Geometry: final body of the model. Coordinates: model frame, mm. A direction names the side the tool comes from. Give positions to 0.01 mm unless a question says otherwise; leave off trailing zeros. Write each loop counter-clockwise with the first axis right and the second up, starting at its lowest first coordinate (ties: lowest second). Pieces come first, ordered by that corner, then holes.
```python
from build123d import *

# Parameters (mm, degrees)
F1_DEPTH     = 12.5
F2_DEPTH     = 12.5
F3_DEPTH     = 12.5
F6_DEPTH     = 7.5
F5_R         = 3.429
F7_DEPTH     = 3
F8_T4_DEPTH  = 66.159380005
F8_S5_R      = 15.125
F8_T6_DEPTH  = 35
F8_T10_DEPTH = 66.159380005
F8_S11_R     = 15.125
F8_T12_DEPTH = 35
F8_T16_DEPTH = 66.159380005
F8_S17_R     = 15.125
F8_T18_DEPTH = 35
F8_T22_DEPTH = 66.159380005
F8_S23_R     = 15.125
F8_T24_DEPTH = 35
F9_T1_DEPTH  = 22.0465191056


# Not quite as in the source:
# - a fillet or chamfer that OpenCascade refuses, or shapes differently, is made with other operations: its cross-section is extruded or revolved along the edge and cut away or added


with BuildPart() as f1:
    # F0 (on Front) → F1 (new body, symmetric)
    with BuildSketch(Plane.XZ):
        with BuildLine():
            Line((-6.3651329838, -12.125), (-6.3651329838, -13.7204485021))
            ThreePointArc((-6.3651329838, -13.7204485021), (0, -15.125), (6.3651329838, -13.7204485021))
            Line((6.3651329838, -13.7204485021), (6.3651329838, -12.125))
            Line((6.3651329838, -12.125), (0, -12.125))
            Line((0, -12.125), (-6.3651329838, -12.125))
        make_face()
        with BuildLine():
            ThreePointArc((6.3651329838, 13.7204485021), (3.2591288258, 14.7696887001), (0, 15.125))
            ThreePointArc((0, 15.125), (-3.2591288258, 14.7696887001), (-6.3651329838, 13.7204485021))
            Line((-6.3651329838, 13.7204485021), (-6.3651329838, 12.125))
            Line((-6.3651329838, 12.125), (0, 12.125))
            Line((0, 12.125), (6.3651329838, 12.125))
            Line((6.3651329838, 12.125), (6.3651329838, 13.7204485021))
        make_face()
        with BuildLine():
            ThreePointArc((15.125, 0), (12.7482991293, 8.1391949424), (6.3651329838, 13.7204485021))
            Line((6.3651329838, 13.7204485021), (6.3651329838, 12.125))
            Line((6.3651329838, 12.125), (0, 12.125))
            ThreePointArc((0, 12.125), (8.5736697219, 8.5736697219), (12.125, 0))
            ThreePointArc((12.125, 0), (8.5736697219, -8.5736697219), (0, -12.125))
            Line((0, -12.125), (6.3651329838, -12.125))
            Line((6.3651329838, -12.125), (6.3651329838, -13.7204485021))
            ThreePointArc((6.3651329838, -13.7204485021), (12.7482991293, -8.1391949424), (15.125, 0))
        make_face()
        with BuildLine():
            Line((-6.3651329838, 12.125), (-6.3651329838, 13.7204485021))
            ThreePointArc((-6.3651329838, 13.7204485021), (-15.125, 0), (-6.3651329838, -13.7204485021))
            Line((-6.3651329838, -13.7204485021), (-6.3651329838, -12.125))
            Line((-6.3651329838, -12.125), (0, -12.125))
            ThreePointArc((0, -12.125), (-12.125, 0), (0, 12.125))
            Line((0, 12.125), (-6.3651329838, 12.125))
        make_face()
    extrude(amount=F1_DEPTH, both=True)

    # F0 (on Front) → F2 (join, through all)
    with BuildSketch(Plane.XZ):
        with BuildLine():
            ThreePointArc((6.3651329838, -13.7204485021), (0, -15.125), (-6.3651329838, -13.7204485021))
            Line((-6.3651329838, -13.7204485021), (-6.3651329838, -54.875))
            Line((-6.3651329838, -54.875), (6.3651329838, -54.875))
            Line((6.3651329838, -54.875), (6.3651329838, -13.7204485021))
        make_face()
    extrude(amount=F2_DEPTH)

    # F0 (on Front) → F3 (join, through all)
    with BuildSketch(Plane.XZ):
        with BuildLine():
            Line((6.3651329838, 15.125), (0, 15.125))
            ThreePointArc((0, 15.125), (3.2591288258, 14.7696887001), (6.3651329838, 13.7204485021))
            Line((6.3651329838, 13.7204485021), (6.3651329838, 15.125))
        make_face()
        with BuildLine():
            Line((0, 15.125), (-6.3651329838, 15.125))
            Line((-6.3651329838, 15.125), (-6.3651329838, 13.7204485021))
            ThreePointArc((-6.3651329838, 13.7204485021), (-3.2591288258, 14.7696887001), (0, 15.125))
        make_face()
    extrude(amount=F3_DEPTH)

    # F4 (on face) → F6 (join)
    with BuildSketch(Plane.XY.offset(15.125)):
        Polygon((1.7145000001, -9.2196011096), (3.4290000001, -6.25), (1.7144999999, -3.2803988905), (-1.7145, -3.2803988907), (-3.4289999999, -6.25), (-1.7145000001, -9.2196011096), align=None)
    extrude(amount=F6_DEPTH)

    # F5 (on face) → F7 (join)
    with BuildSketch(Plane(origin=(0, 0, -54.875), x_dir=(1, 0, 0), z_dir=(0, 0, -1))):
        with Locations((0, 6.2500000003)):
            Circle(F5_R)
    extrude(amount=F7_DEPTH)

    # F8: fillet of radius 5 on 6 edges, made by hand


with BuildPart() as f8_tool2:
    # F8_s3 → F8_t4 (new body)
    with BuildSketch(Plane.XY.offset(-67.3774142536)):
        with BuildLine():
            ThreePointArc((1.3641672983, 0.0004), (4.9006668897, -1.4644660941), (6.3655329838, -5.0009656854))
            Line((6.3655329838, -5.0009656854), (6.8656695523, -5.0009656854))
            ThreePointArc((6.8656695523, -5.0009656854), (6.8652695523, -2.5004828427), (6.8652695523, 0))
            Line((6.8652695523, 0), (6.3651329838, 0.5001365685))
            ThreePointArc((6.3651329838, 0.5001365685), (3.8646501411, 0.5001365685), (1.3641672983, 0.5005365685))
            Line((1.3641672983, 0.5005365685), (1.3641672983, 0.0004))
        make_face()
    extrude(amount=F8_T4_DEPTH)

    # F8_s5 → F8_t6 (cut, symmetric)
    with BuildSketch(Plane.XZ.offset(2.3)):
        Circle(F8_S5_R)
    extrude(amount=F8_T6_DEPTH, both=True, mode=Mode.SUBTRACT)


with BuildPart() as f1_1:
    add(f1.part)

    # F8_t1: cut F8_tool2
    add(f8_tool2.part, mode=Mode.SUBTRACT)


with BuildPart() as f8_tool8:
    # F8_s9 → F8_t10 (new body)
    with BuildSketch(Plane.XY.offset(-1.2180342485)):
        with BuildLine():
            ThreePointArc((-6.3655329838, -5.0009656854), (-4.9006668897, -1.4644660941), (-1.3641672983, 0.0004))
            Line((-1.3641672983, 0.0004), (-1.3641672983, 0.5005365685))
            ThreePointArc((-1.3641672983, 0.5005365685), (-3.8646501411, 0.5001365685), (-6.3651329838, 0.5001365685))
            Line((-6.3651329838, 0.5001365685), (-6.8652695523, 0))
            ThreePointArc((-6.8652695523, 0), (-6.8652695523, -2.5004828427), (-6.8656695523, -5.0009656854))
            Line((-6.8656695523, -5.0009656854), (-6.3655329838, -5.0009656854))
        make_face()
    extrude(amount=-F8_T10_DEPTH)

    # F8_s11 → F8_t12 (cut, symmetric)
    with BuildSketch(Plane.XZ.offset(2.3)):
        Circle(F8_S11_R)
    extrude(amount=F8_T12_DEPTH, both=True, mode=Mode.SUBTRACT)


with BuildPart() as f1_2:
    add(f1_1.part)

    # F8_t7: cut F8_tool8
    add(f8_tool8.part, mode=Mode.SUBTRACT)


with BuildPart() as f8_tool14:
    # F8_s15 → F8_t16 (new body)
    with BuildSketch(Plane.XY.offset(-67.3774142536)):
        with BuildLine():
            ThreePointArc((1.3641672983, -12.5004), (4.9006668897, -11.0355339059), (6.3655329838, -7.4990343146))
            Line((6.3655329838, -7.4990343146), (6.8656695523, -7.4990343146))
            ThreePointArc((6.8656695523, -7.4990343146), (6.8652695523, -9.9995171573), (6.8652695523, -12.5))
            Line((6.8652695523, -12.5), (6.3651329838, -13.0001365685))
            ThreePointArc((6.3651329838, -13.0001365685), (3.8646501411, -13.0001365685), (1.3641672983, -13.0005365685))
            Line((1.3641672983, -13.0005365685), (1.3641672983, -12.5004))
        make_face()
    extrude(amount=F8_T16_DEPTH)

    # F8_s17 → F8_t18 (cut, symmetric)
    with BuildSketch(Plane.XZ.offset(10.2)):
        Circle(F8_S17_R)
    extrude(amount=F8_T18_DEPTH, both=True, mode=Mode.SUBTRACT)


with BuildPart() as f1_3:
    add(f1_2.part)

    # F8_t13: cut F8_tool14
    add(f8_tool14.part, mode=Mode.SUBTRACT)


with BuildPart() as f8_tool20:
    # F8_s21 → F8_t22 (new body)
    with BuildSketch(Plane.XY.offset(-1.2180342485)):
        with BuildLine():
            ThreePointArc((-1.3641672983, -12.5004), (-4.9006668897, -11.0355339059), (-6.3655329838, -7.4990343146))
            Line((-6.3655329838, -7.4990343146), (-6.8656695523, -7.4990343146))
            ThreePointArc((-6.8656695523, -7.4990343146), (-6.8652695523, -9.9995171573), (-6.8652695523, -12.5))
            Line((-6.8652695523, -12.5), (-6.3651329838, -13.0001365685))
            ThreePointArc((-6.3651329838, -13.0001365685), (-3.8646501411, -13.0001365685), (-1.3641672983, -13.0005365685))
            Line((-1.3641672983, -13.0005365685), (-1.3641672983, -12.5004))
        make_face()
    extrude(amount=-F8_T22_DEPTH)

    # F8_s23 → F8_t24 (cut, symmetric)
    with BuildSketch(Plane.XZ.offset(10.2)):
        Circle(F8_S23_R)
    extrude(amount=F8_T24_DEPTH, both=True, mode=Mode.SUBTRACT)


with BuildPart() as f1_4:
    add(f1_3.part)

    # F8_t19: cut F8_tool20
    add(f8_tool20.part, mode=Mode.SUBTRACT)

    # F9: fillet of radius 2 on 2 edges, made by hand

    # F9_s2 → F9_t1 (cut)
    with BuildSketch(Plane.XZ.offset(-4.7732595528)):
        with BuildLine():
            ThreePointArc((-6.3651329838, 13.7204485021), (-5.6409669175, 14.7360395719), (-4.4558291627, 15.125))
            Line((-4.4558291627, 15.125), (-6.3651329838, 15.125))
            Line((-6.3651329838, 15.125), (-6.3651329838, 13.7204485021))
        make_face()
        with BuildLine():
            ThreePointArc((4.4558291627, 15.125), (5.6409669175, 14.7360395719), (6.3651329838, 13.7204485021))
            Line((6.3651329838, 13.7204485021), (6.3651329838, 15.125))
            Line((6.3651329838, 15.125), (4.4558291627, 15.125))
        make_face()
    extrude(amount=F9_T1_DEPTH, mode=Mode.SUBTRACT)


solid = f1_4.part
```
Item 1: Section B-B, the plane x = 8. Return the cut outline in (y, z), plus the area to 3 significant figures.
Found:
outline: (-12.5, -12.84) - (12.5, -12.84) - (12.5, -9.11) - (-12.5, -9.11) - close; (-12.5, 9.11) - (12.5, 9.11) - (12.5, 12.84) - (-12.5, 12.84) - close
area: 186 mm2
Item 2: Line query: L1, parallel to Z at x = -5, y = -4.25 (3 decimals); L2, parallel to Y at x = -1.5, z = -17.5; L3, parallel to X at y = 9, z = -2.5. Output: solid intervals per line, ascending.
Found:
L1: z = -54.875 to -11.046, 11.046 to 15.05
L2: y = -12.5 to 0
L3: x = -14.92 to -11.86, 11.86 to 14.92
Item 3: Section D-D, the plane z = -49. Return the cut outline in (x, y).
Found:
outline: (-6.37, -7.56) arc R5 ccw to (-1.43, -12.5) - (1.43, -12.5) arc R5 ccw to (6.37, -7.56) - (6.37, -4.94) arc R5 ccw to (1.43, 0) - (-1.43, 0) arc R5 ccw to (-6.37, -4.94) - close
Item 4: Section A-A, the plane y = 6.25. Return the cut outline in (x, z) (3 decimals).
Found:
outline: circle Ø30.25 at (0, 0); hole circle Ø24.25 at (0, 0)
Item 5: Reachability of faces 1 (the face through (-6.365, -6, -34)), 2 (the face through (6.365, -6, -35)), 3 (the face through (-2.56, -4.744, 18.822)), 4 (the face through (0, -3.28, 19)) from +Z, -Z, +X, -X, +Y, -Y: full face, straight path, thin tool, end or side. Return the list, or none.
Found:
face 1: -Z, -X, +Y, -Y
face 2: -Z, +X, +Y, -Y
face 3: +Z, -X, +Y
face 4: +Z, +X, -X, +Y
Item 6: Pin query (flat end, axial travel): pin 1 Ø4 at (x, z) = (0.5, 20.5) entering from -Y; pin 2 Ø10 at (x, z) = (5.5, -45.5) entering from -Y; pin 3 Ø1 at (x, z) = (-0.5, 18) entering from +Y; pin 4 Ø6 at (x, y) = (11.5, 1.5) entering from -Z. Return the tip coordinate at first contact, or that it passes through.
Found:
pin 1: stops at y = -9.22
pin 2: stops at y = -12.5
pin 3: stops at y = -3.28
pin 4: stops at z = -12.51
Item 7: Section C-C, the plane z = 9. Return the cut outline in (x, y) (3 decimals), plus the area to 3 significant figures.
Found:
outline: (-12.156, -12.5) - (-8.125, -12.5) - (-8.125, 12.5) - (-12.156, 12.5) - close; (8.125, -12.5) - (12.156, -12.5) - (12.156, 12.5) - (8.125, 12.5) - close
area: 202 mm2
